```python
from build123d import *

# Parameters (mm, degrees)
SKETCH1_R           = 3.175
SKETCH1_R_2         = 0.8
SKETCH1_R_3         = 1.499997
SKETCH1_W           = 6.35
SKETCH1_H           = 12.7
BOSS_EXTRUDE1_DEPTH = 3.175
FILLET1_R           = 3.175
SKETCH2_R           = 1.5
CUT_EXTRUDE1_DEPTH  = 6


with BuildPart() as part:
    # Sketch1 → Boss-Extrude1 (new body, symmetric)
    with BuildSketch(Plane.XY):
        with BuildLine():
            Line((36.576, 9.525), (49.276, 9.525))
            Line((49.276, 9.525), (49.276, -9.525))
            Line((49.276, -9.525), (36.576, -9.525))
            Line((36.576, -9.525), (-64.842812423, -18.25625))
            ThreePointArc((-64.842812423, -18.25625), (-67.372222956, -16.397560002), (-65.861496639, -13.646132709))
            Line((-65.861496639, -13.646132709), (-46.397973184, -6.561989517))
            Line((-46.397973184, -6.561989517), (-36.118832942, 4.353379789))
            ThreePointArc((-36.118832942, 4.353379789), (-34.148654973, 5.769395254), (-31.791214639, 6.343133951))
            Line((-31.791214639, 6.343133951), (36.576, 9.525))
        make_face()
        with Locations((31.496, 0)):
            Circle(SKETCH1_R, mode=Mode.SUBTRACT)
        with Locations((27.606912703, 3.889087297)):
            Circle(SKETCH1_R_2, mode=Mode.SUBTRACT)
        with Locations((35.385087297, -3.889087297)):
            Circle(SKETCH1_R_2, mode=Mode.SUBTRACT)
        with Locations((-31.496, 0)):
            Circle(SKETCH1_R_3, mode=Mode.SUBTRACT)
        with Locations((35.385087297, 3.889087297)):
            Circle(SKETCH1_R_2, mode=Mode.SUBTRACT)
        with Locations((27.606912703, -3.889087297)):
            Circle(SKETCH1_R_2, mode=Mode.SUBTRACT)
        Circle(SKETCH1_R_3, mode=Mode.SUBTRACT)
        with Locations((42.926, 0)):
            Rectangle(SKETCH1_W, SKETCH1_H, mode=Mode.SUBTRACT)
    extrude(amount=BOSS_EXTRUDE1_DEPTH, both=True)

    # Fillet1
    fillet1_edges = [part.edges().sort_by_distance(p)[0] for p in [
        (49.276, 9.525, 0),
        (49.276, -9.525, 0),
    ]]
    fillet(fillet1_edges, radius=FILLET1_R)

    # Sketch2 → Cut-Extrude1 (cut)
    with BuildSketch(Plane(origin=(-3.318549049, 9.117638577, 0), x_dir=(0.939692621, 0.342020143, 0), z_dir=(-0.342020143, 0.939692621, 0))):
        with Locations((-49.019165615, 0)):
            Circle(SKETCH2_R)
    extrude(amount=-CUT_EXTRUDE1_DEPTH, mode=Mode.SUBTRACT)


solid = part.part
```
Work out the finished part from the listing and answer in its coordinate system (mm). A direction names the side the tool comes from. Give positions to 0.01 mm unless a question says otherwise; leave off trailing zeros. Write each loop counter-clockwise with the first axis right and the second up, starting at its lowest first coordinate (ties: lowest second). Pieces come first, ordered by that corner, then holes. Notation, with made-up numbers: (19, 83.5) -> (26, 83.5) arc R22 cw to (26, 109.5) -> close; hole circle Ø2 at (27.5, 34). An arc over 180 degrees is marked (long way). Write item = value, one per line.
Q1. A tool of negligible diameter and unlimited length cuts with its end or side. For faces 4 (the flat face through (-41.33, -1.18, 0.04)), 5 (the flat face through (43, 6.35, 0)), 6 (the flat face through (41, -9.525, 0)), from which of +Z, -Z, +X, -X, +Y, -Y can it reach the whole face along a straight path? Write none if from no direction.
Computed values:
face_4 = +Z, -Z, -X, +Y
face_5 = +Z, -Z
face_6 = +Z, -Z, +X, -Y
Q2. Section C-C on x = 0 is taken. Determine the outline of the cut face in (y, z) (3 decimals), and give its area (3 significant figures).
Computed values:
outline = (-12.674, -3.175) -> (-1.5, -3.175) -> (-1.5, 3.175) -> (-12.674, 3.175) -> close; (1.5, -3.175) -> (7.823, -3.175) -> (7.823, 3.175) -> (1.5, 3.175) -> close
area = 111 mm^2
Q3. Consider line 1 along Y through (x, z) = (41.5, 1.75) (3 decimals); line 2 along X through (y, z) = (-4, -2.5); line 3 along X through (y, z) = (-2.5, -1). Determine where each line is inside the solid, lowest interval first.
Computed values:
line_1 = -9.525 to -6.35, 6.35 to 9.525
line_2 = -43.99 to 26.81, 28.4 to 34.59, 36.18 to 39.75, 46.1 to 49.28
line_3 = -42.57 to 29.54, 33.45 to 39.75, 46.1 to 49.28
Q4. Section A-A on x = 41 is taken. Determine the outline of the cut face in (y, z) (3 decimals).
Computed values:
outline = (-9.525, -3.175) -> (-6.35, -3.175) -> (-6.35, 3.175) -> (-9.525, 3.175) -> close; (6.35, -3.175) -> (9.525, -3.175) -> (9.525, 3.175) -> (6.35, 3.175) -> close
Q5. Flat-ended cylindrical pins translate along their axes: pin 1 Ø1.5 at (x, z) = (-34, -1.5) entering from -Y; pin 2 Ø2.5 at (x, y) = (27.61, 3.89) entering from +Z (3 decimals); pin 3 Ø1.5 at (x, z) = (-15, -0.5) entering from -Y; pin 4 Ø1.5 at (x, z) = (-39.5, -2) entering from +Y. Find the tip coordinate at first contact, or state that the pin passes through.
Computed values:
pin_1 = -15.67
pin_2 = 3.175
pin_3 = -14.03
pin_4 = 1.56
Q6. Section D-D on x = -34 is taken. Determine the outline of the cut face in (y, z) (3 decimals).
Computed values:
outline = (-15.601, -3.175) -> (5.835, -3.175) -> (5.835, 3.175) -> (-15.601, 3.175) -> close
Q7. Section B-B on y = 0 is taken. Determine the outline of the cut face in (x, z) (3 decimals), and give its area (3 significant figures).
Computed values:
outline = (-40.218, -3.175) -> (-32.996, -3.175) -> (-32.996, 3.175) -> (-40.218, 3.175) -> close; (-29.996, -3.175) -> (-1.5, -3.175) -> (-1.5, 3.175) -> (-29.996, 3.175) -> close; (1.5, -3.175) -> (28.321, -3.175) -> (28.321, 3.175) -> (1.5, 3.175) -> close; (34.671, -3.175) -> (39.751, -3.175) -> (39.751, 3.175) -> (34.671, 3.175) -> close; (46.101, -3.175) -> (49.276, -3.175) -> (49.276, 3.175) -> (46.101, 3.175) -> close
area = 450 mm^2
Q8. For a pull along Y with two mould halves and no side action, classify faces 1 (the flat face through (49.276, 0, 0)), 2 (the flat face through (1.91, 7.91, 0.04)), 3 (the flat face through (39.751, 0, 0)) as pulls with the +Y half, pulls with the -Y half, needs draft (parallel to the pull), parting line crosses it, or undercut.
Computed values:
face_1 = needs draft
face_2 = pulls with the +Y half
face_3 = undercut
